CAD build for the part. Positions are in the model's coordinates, mm. A direction names the side the tool comes from. Round coordinates to 2 decimals unless told otherwise and drop trailing zeros. Write each loop counter-clockwise with the first axis right and the second up, starting at its lowest first coordinate (ties: lowest second). Pieces come first, ordered by that corner, then holes. Notation, with made-up numbers: (77, 39.5) - (107, 39.5) arc R14 cw to (107, 53.5) - close; hole circle Ø2 at (20, 83). An arc over 180 degrees is marked (long way). Answer in a Markdown table with one row per item.
```python
from build123d import *

# Parameters (mm, degrees)
SKETCH1_W           = 74.93
SKETCH1_H           = 30.48
SKETCH1_R           = 1.905
BOSS_EXTRUDE1_DEPTH = 1.5748
SKETCH2_W           = 25
SKETCH2_H           = 7.5
BOSS_EXTRUDE2_DEPTH = 5.08
CUT_EXTRUDE1_START  = -1.016
SKETCH3_W           = 25
SKETCH3_H           = 15
SKETCH3_W_2         = 23
SKETCH3_H_2         = 13
CUT_EXTRUDE1_DEPTH  = 4.064
SKETCH4_W           = 8.5
SKETCH4_H           = 5
BOSS_EXTRUDE3_DEPTH = 1.524
SKETCH5_W           = 1
SKETCH5_H           = 5
BOSS_EXTRUDE4_DEPTH = 2.286


with BuildPart() as part:
    # Sketch1 → Boss-Extrude1 (new body)
    with BuildSketch(Plane(origin=(0, 0, 0), x_dir=(1, 0, 0), z_dir=(0, 1, 0))):
        Rectangle(SKETCH1_W, SKETCH1_H)
        with Locations((-34.925, 12.7)):
            Circle(SKETCH1_R, mode=Mode.SUBTRACT)
        with Locations((34.925, 12.7)):
            Circle(SKETCH1_R, mode=Mode.SUBTRACT)
        with Locations((-34.925, -12.7)):
            Circle(SKETCH1_R, mode=Mode.SUBTRACT)
        with Locations((34.925, -12.7)):
            Circle(SKETCH1_R, mode=Mode.SUBTRACT)
    extrude(amount=-BOSS_EXTRUDE1_DEPTH)

    # Sketch2 → Boss-Extrude2 (add)
    with BuildSketch(Plane(origin=(0, 0, 0), x_dir=(1, 0, 0), z_dir=(0, 1, 0))):
        with Locations((-24.33, 3.75)):
            Rectangle(SKETCH2_W, SKETCH2_H)
        with Locations((-24.33, -3.75)):
            Rectangle(SKETCH2_W, SKETCH2_H)
    extrude(amount=BOSS_EXTRUDE2_DEPTH)

    # Sketch3 → Cut-Extrude1 (cut)
    with BuildSketch(Plane(origin=(0, 5.08, 0), x_dir=(1, 0, 0), z_dir=(0, 1, 0)).offset(CUT_EXTRUDE1_START)):
        with Locations((-24.33, 0)):
            Rectangle(SKETCH3_W, SKETCH3_H)
        with Locations((-24.33, 0)):
            Rectangle(SKETCH3_W_2, SKETCH3_H_2, mode=Mode.SUBTRACT)
    extrude(amount=-CUT_EXTRUDE1_DEPTH, mode=Mode.SUBTRACT)

    # Sketch4 → Boss-Extrude3 (add)
    with BuildSketch(Plane(origin=(0, 5.08, 0), x_dir=(1, 0, 0), z_dir=(0, 1, 0))):
        with Locations((-29.58, 0)):
            Rectangle(SKETCH4_W, SKETCH4_H)
    extrude(amount=BOSS_EXTRUDE3_DEPTH)

    # Sketch5 → Boss-Extrude4 (add)
    with BuildSketch(Plane(origin=(0, 6.604, 0), x_dir=(1, 0, 0), z_dir=(0, 1, 0))):
        with Locations((-33.33, 0)):
            Rectangle(SKETCH5_W, SKETCH5_H)
    extrude(amount=BOSS_EXTRUDE4_DEPTH)


solid = part.part
```
Q1. Saw through at A-A on z = -12.7. List the corners of the cut face in (x, y) (3 decimals).
Computed:
| item | result |
|---|---|
| outline | (-37.465, -1.575) - (-36.83, -1.575) - (-36.83, 0) - (-37.465, 0) - close; (-33.02, -1.575) - (33.02, -1.575) - (33.02, 0) - (-33.02, 0) - close; (36.83, -1.575) - (37.465, -1.575) - (37.465, 0) - (36.83, 0) - close |
Q2. Flat gauge pins, fed straight in: pin 1 (3.5 mm diameter, centred on y = 2.5, z = 2.5, fed in from +X); pin 2 (3 mm diameter, centred on y = 2.5, z = -4.5, fed in from +X); pin 3 (1.7 mm diameter, centred on y = 6, z = 1, fed in from +X); pin 4 (5 mm diameter, centred on y = 6, z = -11.5, fed in from +X). Where does each tip first touch, or does it go through?
Computed:
| item | result |
|---|---|
| pin 1 | stops at x = -11.83 |
| pin 2 | stops at x = -12.83 |
| pin 3 | stops at x = -25.33 |
| pin 4 | passes through |
Q3. Pull direction Y, two halves, no side cores. Call faces 5 (the flat face through (-25, 4.064, 7)), 6 (the flat face through (-32.83, 8, 0)), 7 (the flat face through (-29, 6.604, 0)): released by +Y, released by -Y, zero draft, split by the parting line, or undercut.
Computed:
| item | result |
|---|---|
| face 5 | undercut |
| face 6 | zero draft |
| face 7 | released by +Y |
Q4. Saw through at D-D on y = 2.5. List the corners of the cut face in (x, z), then the cut area to 3 significant figures.
Computed:
| item | result |
|---|---|
| outline | (-35.83, -6.5) - (-12.83, -6.5) - (-12.83, 6.5) - (-35.83, 6.5) - close |
| area | 299 mm2 |
Q5. Saw through at C-C on z = -3.5. List the corners of the cut face in (x, y) (3 decimals).
Computed:
| item | result |
|---|---|
| outline | (-37.465, -1.575) - (37.465, -1.575) - (37.465, 0) - (-12.83, 0) - (-12.83, 4.064) - (-11.83, 4.064) - (-11.83, 5.08) - (-36.83, 5.08) - (-36.83, 4.064) - (-35.83, 4.064) - (-35.83, 0) - (-37.465, 0) - close |
Q6. Drill centre lines: line 1 (X direction, y = -1.15, z = -12.7) (3 decimals); line 2 (Y direction, x = 27.5, z = 8.5); line 3 (Z direction, x = -29, y = 6.5). Where is each one in solid material? Low to high.
Computed:
| item | result |
|---|---|
| line 1 | x = -37.465 to -36.83, -33.02 to 33.02, 36.83 to 37.465 |
| line 2 | y = -1.57 to 0 |
| line 3 | z = -2.5 to 2.5 |
Q7. Saw through at B-B on x = -24.5. List the corners of the cut face in (y, z).
Computed:
| item | result |
|---|---|
| outline | (-1.57, -15.24) - (0, -15.24) - (0, -6.5) - (4.06, -6.5) - (4.06, -7.5) - (5.08, -7.5) - (5.08, 7.5) - (4.06, 7.5) - (4.06, 6.5) - (0, 6.5) - (0, 15.24) - (-1.57, 15.24) - close |
Q8. 3-axis set-ups, long thin cutter, end or side, ignore diameter. For faces 1 (the flat face through (-35.83, 2, 0)), 2 (the flat face through (-30, 6, 2.5)), 3 (the flat face through (-24, 2, -6.5)), 4 (the flat face through (-25.33, 6, 0)): which of +Z, -Z, +X, -X, +Y, -Y reach the whole face in a straight line?
Computed:
| item | result |
|---|---|
| face 1 | +Z, -Z, -X |
| face 2 | +Z, +X, -X, +Y |
| face 3 | -Z, +X, -X |
| face 4 | +Z, -Z, +X, +Y |
